from build123d import *

# Parameters (mm, degrees)
SKETCH1_R           = 2.65
BOSS_EXTRUDE1_DEPTH = 6.35
SKETCH2_R           = 3.555
SKETCH2_R_2         = 2.65
BOSS_EXTRUDE2_DEPTH = 2.5


with BuildPart() as part:
    # Sketch1 → Boss-Extrude1 (new body)
    with BuildSketch(Plane(origin=(0, 0, 0), x_dir=(1, 0, 0), z_dir=(0, 1, 0))):
        Polygon((4.21, 2.886751346), (-0.79, 5.773502692), (-5.79, 2.886751346), (-5.79, -2.886751346), (-0.79, -5.773502692), (4.21, -2.886751346), (4.21, -1), (4.06, -1), (4.06, 1), (4.21, 1), align=None)
        Circle(SKETCH1_R, mode=Mode.SUBTRACT)
    extrude(amount=BOSS_EXTRUDE1_DEPTH)

    # Sketch2 → Boss-Extrude2 (add)
    with BuildSketch(Plane(origin=(0, 6.35, 0), x_dir=(1, 0, 0), z_dir=(0, 1, 0))):
        with Locations((-0.79, 0)):
            Circle(SKETCH2_R)
        Circle(SKETCH2_R_2, mode=Mode.SUBTRACT)
    extrude(amount=BOSS_EXTRUDE2_DEPTH)


solid = part.part
Check sheet for the modelled part. Datum: model origin and axes. Units: mm. A direction names the side the tool comes from. Round coordinates to 2 decimals unless told otherwise and drop trailing zeros. Write each loop counter-clockwise with the first axis right and the second up, starting at its lowest first coordinate (ties: lowest second). Pieces come first, ordered by that corner, then holes. Notation, with made-up numbers: (30.25, 52.25) -> (57.25, 52.25) arc R24 cw to (57.25, 80.25) -> close; hole circle Ø2 at (34, 89.25). An arc over 180 degrees is marked (long way). Answer as CSV lines item,"result". Start each with the question number.
1) Section check B-B on y = 1. Enter the section's corners in (x, z), and give its area (3 significant figures).
2) Release check for a two-part mould opening along Z. For faces 4 (the flat face through (1.675, 3.131, 4.35)), 5 (the flat face through (-5.79, 3, 0)), 6 (the cylindrical face through (2.45, 4.36, 1.01)) record: pulls with the +Z half, pulls with the -Z half, needs draft (parallel to the pull), parting line crosses it, or undercut.
3) Tool access check on faces 1 (the flat face through (-3.325, 3.131, 4.31)), 2 (the flat face through (-1, 6.35, 4)), 3 (the flat face through (4.06, 3, 0)). Record the directions out of +Z, -Z, +X, -X, +Y, -Y that give a thin tool (end or side, any length) a straight path to the whole face; none if there is none.
4) Section check A-A on z = 0. Enter the section's corners in (x, y) (3 decimals).
5) Material ranges on line 1 (X direction, y = 5.75, z = 0); line 2 (Y direction, x = 3.25, z = -0.5); line 3 (X direction, y = 1.5, z = -2.25), recorded low to high. Write a range as from..to.
6) Section check C-C on x = 0.25. Enter the section's corners in (y, z), and give its area (3 significant figures).
7) Go/stop test with flat-tipped pins: P1, Ø1, axis at y = 3, z = 0, coming from the +X side; P2, Ø1, axis at x = -2, z = -0.5, coming from the +Y side; P3, Ø1, axis at x = 0.5, y = 4, coming from the +Z side; P4, Ø1.5, axis at x = 3, y = 2.5, coming from the +Z side. Record where each tip stops, or that it passes through.
8) Section check D-D on x = -3.5. Enter the section's corners in (y, z), and give its area (3 significant figures).
Found:
1,outline,"(-5.79, -2.89) -> (-0.79, -5.77) -> (4.21, -2.89) -> (4.21, -1) -> (4.06, -1) -> (4.06, 1) -> (4.21, 1) -> (4.21, 2.89) -> (-0.79, 5.77) -> (-5.79, 2.89) -> close; hole circle Ø5.3 at (0, 0)"
1,area,"64.2 mm^2"
2,face 4,"pulls with the +Z half"
2,face 5,"needs draft"
2,face 6,"undercut"
3,face 1,"+Z, -X, +Y, -Y"
3,face 2,"+Y"
3,face 3,"+X, +Y, -Y"
4,outline,"(-5.79, 0) -> (-2.65, 0) -> (-2.65, 8.85) -> (-4.345, 8.85) -> (-4.345, 6.35) -> (-5.79, 6.35) -> close; (2.65, 0) -> (4.06, 0) -> (4.06, 6.35) -> (2.765, 6.35) -> (2.765, 8.85) -> (2.65, 8.85) -> close"
5,line 1,"x = -5.79..-2.65, 2.65..4.06"
5,line 2,"y = 0..6.35"
5,line 3,"x = -5.79..-1.4, 1.4..4.21"
6,outline,"(0, -5.17) -> (6.35, -5.17) -> (6.35, -3.4) -> (8.85, -3.4) -> (8.85, -2.64) -> (0, -2.64) -> close; (0, 2.64) -> (8.85, 2.64) -> (8.85, 3.4) -> (6.35, 3.4) -> (6.35, 5.17) -> (0, 5.17) -> close"
6,area,"36.0 mm^2"
7,P1,"stops at x = 4.06"
7,P2,"passes through"
7,P3,"stops at z = 5.32"
7,P4,"stops at z = 4.02"
8,outline,"(0, -4.21) -> (6.35, -4.21) -> (6.35, -2.3) -> (8.85, -2.3) -> (8.85, 2.3) -> (6.35, 2.3) -> (6.35, 4.21) -> (0, 4.21) -> close"
8,area,"65.0 mm^2"
